from build123d import *

# Parameters (mm, degrees)
BASE_FLANGE1_DEPTH  = 76.2
CUT_EXTRUDE1_DEPTH  = 1.5875
CUT_EXTRUDE4_DEPTH  = 223.428182145
SKETCH11_W          = 15.875
SKETCH11_H          = 1.5875
BOSS_EXTRUDE1_DEPTH = 25.4
SKETCH12_W          = 15.875
SKETCH12_H          = 1.5875
BOSS_EXTRUDE2_DEPTH = 25.4
SKETCH13_R          = 2.54
CUT_EXTRUDE5_DEPTH  = 25.4
SKETCH14_R          = 2.54
CUT_EXTRUDE6_DEPTH  = 25.4
SKETCH15_R          = 2.54
CUT_EXTRUDE7_DEPTH  = 25.4


# Sheet-metal steps are written as plain solids
with BuildPart() as part:
    # Sketch1 → Base-Flange1 (new, symmetric)
    with BuildSketch(Plane(origin=(0, 0, 0), x_dir=(1, 0, 0), z_dir=(0, 1, 0))):
        with BuildLine():
            Line((-111.125, -40.005), (-95.25, -40.005))
            ThreePointArc((-95.25, -40.005), (-93.00493597, -39.07506403), (-92.075, -36.83))
            Line((-92.075, -36.83), (-92.075, 38.4175))
            ThreePointArc((-92.075, 38.4175), (-91.610032015, 39.540032015), (-90.4875, 40.005))
            Line((-90.4875, 40.005), (90.4875, 40.005))
            ThreePointArc((90.4875, 40.005), (91.610032015, 39.540032015), (92.075, 38.4175))
            Line((92.075, 38.4175), (92.075, -36.83))
            ThreePointArc((92.075, -36.83), (93.00493597, -39.07506403), (95.25, -40.005))
            Line((95.25, -40.005), (111.125, -40.005))
            Line((111.125, -40.005), (111.125, -38.4175))
            Line((111.125, -38.4175), (95.25, -38.4175))
            ThreePointArc((95.25, -38.4175), (94.127467985, -37.952532015), (93.6625, -36.83))
            Line((93.6625, -36.83), (93.6625, 38.4175))
            ThreePointArc((93.6625, 38.4175), (92.73256403, 40.66256403), (90.4875, 41.5925))
            Line((90.4875, 41.5925), (-90.4875, 41.5925))
            ThreePointArc((-90.4875, 41.5925), (-92.73256403, 40.66256403), (-93.6625, 38.4175))
            Line((-93.6625, 38.4175), (-93.6625, -36.83))
            ThreePointArc((-93.6625, -36.83), (-94.127467985, -37.952532015), (-95.25, -38.4175))
            Line((-95.25, -38.4175), (-111.125, -38.4175))
            Line((-111.125, -38.4175), (-111.125, -40.005))
        make_face()
    extrude(amount=BASE_FLANGE1_DEPTH, both=True)

    # Sketch6 → Cut-Extrude1 (cut)
    with BuildSketch(Plane.XY.offset(-40.005)):
        with BuildLine():
            Line((-55.5625, -50.8), (55.5625, -50.8))
            ThreePointArc((55.5625, -50.8), (60.052628061, -48.940128061), (61.9125, -44.45))
            Line((61.9125, -44.45), (61.9125, 44.45))
            ThreePointArc((61.9125, 44.45), (60.052628061, 48.940128061), (55.5625, 50.8))
            Line((55.5625, 50.8), (-55.5625, 50.8))
            ThreePointArc((-55.5625, 50.8), (-60.052628061, 48.940128061), (-61.9125, 44.45))
            Line((-61.9125, 44.45), (-61.9125, -44.45))
            ThreePointArc((-61.9125, -44.45), (-60.052628061, -48.940128061), (-55.5625, -50.8))
        make_face()
    extrude(amount=-CUT_EXTRUDE1_DEPTH, mode=Mode.SUBTRACT)

    # Sketch10 → Cut-Extrude4 (cut, through all)
    with BuildSketch(Plane.ZY.offset(93.6625)):
        with BuildLine():
            Line((12.060895861, 43.449063634), (30.48, 11.848349253))
            Line((30.48, 11.848349253), (30.48, 69.5325))
            ThreePointArc((30.48, 69.5325), (30.015032015, 70.655032015), (28.8925, 71.12))
            Line((28.8925, 71.12), (13.49375, 71.12))
            ThreePointArc((13.49375, 71.12), (12.371217985, 70.655032015), (11.90625, 69.5325))
            Line((11.90625, 69.5325), (11.90625, 44.1325))
            ThreePointArc((11.90625, 44.1325), (11.945394066, 43.782142822), (12.060895861, 43.449063634))
        make_face()
        with BuildLine():
            Line((-13.49375, 71.12), (-28.8925, 71.12))
            ThreePointArc((-28.8925, 71.12), (-30.015032015, 70.655032015), (-30.48, 69.5325))
            Line((-30.48, 69.5325), (-30.48, 11.848349253))
            Line((-30.48, 11.848349253), (-12.060895861, 43.449063634))
            ThreePointArc((-12.060895861, 43.449063634), (-11.945394066, 43.782142822), (-11.90625, 44.1325))
            Line((-11.90625, 44.1325), (-11.90625, 69.5325))
            ThreePointArc((-11.90625, 69.5325), (-12.371217985, 70.655032015), (-13.49375, 71.12))
        make_face()
        with BuildLine():
            Line((30.48, -69.5325), (30.48, -11.848349253))
            Line((30.48, -11.848349253), (12.060895861, -43.449063634))
            ThreePointArc((12.060895861, -43.449063634), (11.945394066, -43.782142822), (11.90625, -44.1325))
            Line((11.90625, -44.1325), (11.90625, -69.5325))
            ThreePointArc((11.90625, -69.5325), (12.371217985, -70.655032015), (13.49375, -71.12))
            Line((13.49375, -71.12), (28.8925, -71.12))
            ThreePointArc((28.8925, -71.12), (30.015032015, -70.655032015), (30.48, -69.5325))
        make_face()
        with BuildLine():
            Line((-12.060895861, -43.449063634), (-30.48, -11.848349253))
            Line((-30.48, -11.848349253), (-30.48, -69.5325))
            ThreePointArc((-30.48, -69.5325), (-30.015032015, -70.655032015), (-28.8925, -71.12))
            Line((-28.8925, -71.12), (-13.49375, -71.12))
            ThreePointArc((-13.49375, -71.12), (-12.371217985, -70.655032015), (-11.90625, -69.5325))
            Line((-11.90625, -69.5325), (-11.90625, -44.1325))
            ThreePointArc((-11.90625, -44.1325), (-11.945394066, -43.782142822), (-12.060895861, -43.449063634))
        make_face()
    extrude(amount=-CUT_EXTRUDE4_DEPTH, mode=Mode.SUBTRACT)

    # Sketch11 → Boss-Extrude1 (add)
    with BuildSketch(Plane.XZ.offset(76.2)):
        with Locations((103.1875, 39.21125)):
            Rectangle(SKETCH11_W, SKETCH11_H)
    extrude(amount=BOSS_EXTRUDE1_DEPTH)

    # Sketch12 → Boss-Extrude2 (add)
    with BuildSketch(Plane(origin=(0, -76.2, 0), x_dir=(-1, 0, 0), z_dir=(0, -1, 0))):
        with Locations((103.1875, -39.21125)):
            Rectangle(SKETCH12_W, SKETCH12_H)
    extrude(amount=BOSS_EXTRUDE2_DEPTH)

    # Sketch13 → Cut-Extrude5 (cut)
    with BuildSketch(Plane(origin=(0, 0, 38.4175), x_dir=(-1, 0, 0), z_dir=(0, 0, -1))):
        with Locations((-102.87, -88.9)):
            Circle(SKETCH13_R)
        with Locations((-103.505, 63.5)):
            Circle(SKETCH13_R)
    extrude(amount=-CUT_EXTRUDE5_DEPTH, mode=Mode.SUBTRACT)

    # Sketch14 → Cut-Extrude6 (cut)
    with BuildSketch(Plane(origin=(0, 0, 38.4175), x_dir=(-1, 0, 0), z_dir=(0, 0, -1))):
        with Locations((103.505, 63.5)):
            Circle(SKETCH14_R)
    extrude(amount=-CUT_EXTRUDE6_DEPTH, mode=Mode.SUBTRACT)

    # Sketch15 → Cut-Extrude7 (cut)
    with BuildSketch(Plane(origin=(0, 0, 38.4175), x_dir=(-1, 0, 0), z_dir=(0, 0, -1))):
        with Locations((102.87, -88.9)):
            Circle(SKETCH15_R)
    extrude(amount=-CUT_EXTRUDE7_DEPTH, mode=Mode.SUBTRACT)


solid = part.part
Design review of the part built by this model. Coordinates are the model's own, in mm. A direction names the side the tool comes from. Round coordinates to 2 decimals unless told otherwise and drop trailing zeros. Loops run counter-clockwise (first coordinate to the right, second up) from the corner with the lowest first, then second, coordinate; pieces in that order, holes last. Notation, with made-up numbers: (66, 68) -> (100, 68) arc R12 ccw to (100, 75) -> close; hole circle Ø3 at (10.25, 86.5). An arc over 180 degrees is marked (long way). Use one line per item in the form item = value. Start each with the question number.
Q1. Machinability: for faces 4 (the face through (1, 52, -41.592)), 5 (the face through (103, -11, 38.418)), 6 (the face through (-60.1, -48.89, -40.79)), 7 (the face through (92.86, 27.43, -21.4)), 8 (the face through (-1, 52, -40.005)), which of the approach directions +Z, -Z, +X, -X, +Y, -Y give a long, thin tool a straight path to every point of the face, cutting with its end or side? Answer none if there is none.
Q2. Draft analysis for pull direction X (two halves, no side actions). For faces 1 (the face through (-103, -11, 40.005)), 2 (the face through (60, -48.99, -40.79)), 3 (the face through (-93.662, 1, -1)), state which applies: +X half, -X half, draft (parallel to the pull), parting line (faces both ways), or undercut.
Q3. We need section C-C on z = -33. Give the boundary of the cut face in (x, y) (1 decimal), then the cut area to 3 significant figures.
Q4. We need section B-B on y = -88.9. State how many separate pieces and enclosed holes the cut face has, then the cut area to 3 significant figures.
Q5. For pin 1 Ø0.5 at (x, y) = (-93, -63) entering from -Z (3 decimals); pin 2 Ø10 at (y, z) = (9.5, 30.5) entering from -X; pin 3 Ø0.8 at (x, y) = (93, 31.5) entering from -Z; pin 4 Ø4 at (x, y) = (102.87, -88.9) entering from -Z, all flat-tipped, find the tip position at first contact; note any pin that passes through.
Q6. Wall thickness on line 1 along X through (y, z) = (-33, 4) (1 decimal); line 2 along Y through (x, z) = (102, 39); line 3 along X through (y, z) = (-88, 39) (3 decimals): over which ranges is each line inside the solid? List them lowest first. Write a range as [from, to].
Q7. We need section A-A on x = -30. Give the boundary of the cut face in (y, z) (1 decimal).
Calculated:
q1.face_4 = -Z, +X, -X, +Y, -Y
q1.face_5 = -Z, +X, +Y, -Y
q1.face_6 = +Z, -Z
q1.face_7 = +X, -X
q1.face_8 = +Z, +Y, -Y
q2.face_1 = draft
q2.face_2 = undercut
q2.face_3 = -X half
q3.outline = (-93.7, -76.2) -> (-92.1, -76.2) -> (-92.1, 76.2) -> (-93.7, 76.2) -> close; (92.1, -76.2) -> (93.7, -76.2) -> (93.7, 76.2) -> (92.1, 76.2) -> close
q3.area = 484 mm²
q4.separate_pieces = 4
q4.enclosed_holes = 0
q4.area = 34.3 mm²
q5.pin_1 = -40.645
q5.pin_2 = -93.66
q5.pin_3 = -40.79
q5.pin_4 = through
q6.line_1 = [-93.7, -92.1], [92.1, 93.7]
q6.line_2 = [-101.6, -91.29], [-86.51, 61.45], [65.55, 76.2]
q6.line_3 = [-111.125, -105.245], [-100.495, -95.25], [95.25, 100.495], [105.245, 111.125]
q7.outline = (-76.2, -41.6) -> (-50.8, -41.6) -> (-50.8, -40) -> (-76.2, -40) -> close; (50.8, -41.6) -> (76.2, -41.6) -> (76.2, -40) -> (50.8, -40) -> close
